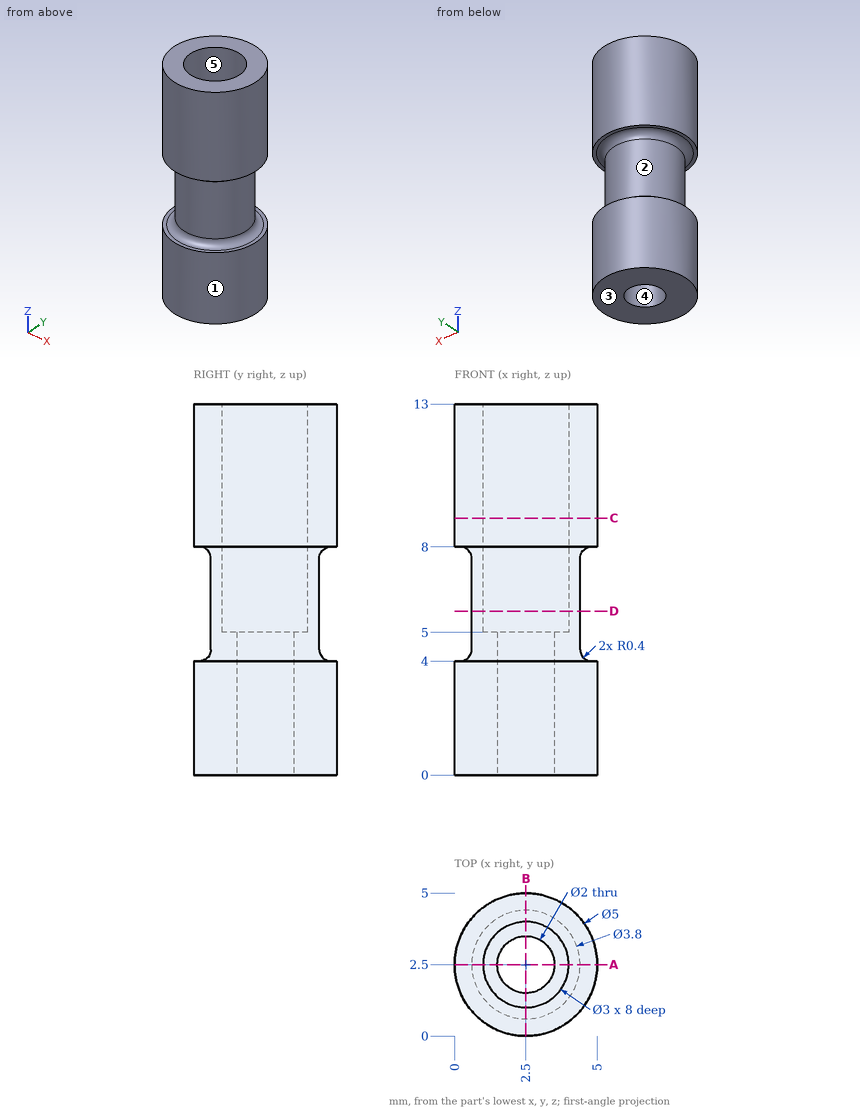
Geometry: see drawing. Coordinates: mm, zero at the bounding-box minimum. A direction names the side the tool comes from. Round coordinates to 2 decimals unless told otherwise and drop trailing zeros. Loops run counter-clockwise (first coordinate to the right, second up) from the corner with the lowest first, then second, coordinate; pieces in that order, holes last. Notation, with made-up numbers: M -2,-33 L 38,-33 A20 cw 38,-10 Z; hole C -4,16.25 d8. An arc over 180 degrees is marked long. Use a Markdown table: item, result. Add a question column.
1. Pull-direction query (Z, two-part tool) for the marked faces 1, 2 and 3; classes: +Z half, -Z half, draft (parallel to the pull), parting line (faces both ways), or undercut.
2. Set-up query: the marked faces 4 and 5. Return all of +Z, -Z, +X, -X, +Y, -Y with unobstructed straight access to the full face (end or side cutting, diameter ignored); none if empty.
3. Contact query for flat-ended pins moving along their axis: pin 1 (1.2 mm diameter, centred on x = 2.5, y = 2.5, fed in from -Z); pin 2 (2.5 mm diameter, centred on x = 2.5, y = 2.5, fed in from +Z). Output: stop coordinate, or through.
4. Cut plane D-D, the plane z = 5.75. Output: boundary loops of the cut face in (x, y), and give its area (3 significant figures).
5. Cut plane C-C, the plane z = 9. Output: boundary loops of the cut face in (x, y), and give its area (3 significant figures).
6. Ray query, line 1 along Y through (x, z) = (2.5, 9.5); line 2 along Y through (x, z) = (2.5, 3.4); line 3 along Z through (x, y) = (4.75, 2.55). Return the intervals inside material, ascending. Write a range as [from, to].
7. Cut plane A-A, the plane y = 2.5. Output: boundary loops of the cut face in (x, z).
Solution:
| question | item | result |
|---|---|---|
| 1 | face 1 | draft |
| 1 | face 2 | undercut |
| 1 | face 3 | -Z half |
| 2 | face 4 | +Z, -Z |
| 2 | face 5 | +Z |
| 3 | pin 1 | passes through |
| 3 | pin 2 | stops at z = 5 |
| 4 | outline | C 2.5,2.5 d3.8; hole C 2.5,2.5 d3 |
| 4 | area | 4.27 mm2 |
| 5 | outline | C 2.5,2.5 d5; hole C 2.5,2.5 d3 |
| 5 | area | 12.6 mm2 |
| 6 | line 1 | y = [0, 1], [4, 5] |
| 6 | line 2 | y = [0, 1.5], [3.5, 5] |
| 6 | line 3 | z = [0, 4], [8, 13] |
| 7 | outline | M 0,0 L 1.5,0 L 1.5,5 L 1,5 L 1,13 L 0,13 L 0,8 L 0.2,8 A0.4 cw 0.6,7.6 L 0.6,4.4 A0.4 cw 0.2,4 L 0,4 Z; M 3.5,0 L 5,0 L 5,4 L 4.8,4 A0.4 cw 4.4,4.4 L 4.4,7.6 A0.4 cw 4.8,8 L 5,8 L 5,13 L 4,13 L 4,5 L 3.5,5 Z |
